Input: part model. Units: mm. Frame: model coordinates. A direction names the side the tool comes from. Round coordinates to 2 decimals unless told otherwise and drop trailing zeros. Order: outer loops, then holes, each group sorted by start corner. A loop starts at its lowest first (then second) coordinate and runs counter-clockwise, first axis right, second up. Notation, with made-up numbers: (71, 21) -> (130, 21) arc R17 cw to (130, 54) -> close; hole circle Ø3 at (-1.5, 43.5). An arc over 180 degrees is marked (long way). Use a Markdown table: item, result.
from build123d import *

# Parameters (mm, degrees)
SKETCH1_R           = 1.2
BOSS_EXTRUDE1_DEPTH = 8.7
CUT_EXTRUDE2_DEPTH  = 3
CUT_EXTRUDE3_DEPTH  = 3.8
CUT_EXTRUDE4_DEPTH  = 1.9
SKETCH5_W           = 1
SKETCH5_H           = 1.5
CUT_EXTRUDE5_DEPTH  = 3
FILLET1_R           = 1


with BuildPart() as part:
    # Sketch1 → Boss-Extrude1 (new body)
    with BuildSketch(Plane.XY):
        with BuildLine():
            Line((21.25, -19.25), (21.25, 19.25))
            ThreePointArc((21.25, 19.25), (20.664213562, 20.664213562), (19.25, 21.25))
            Line((19.25, 21.25), (-19.25, 21.25))
            ThreePointArc((-19.25, 21.25), (-20.664213562, 20.664213562), (-21.25, 19.25))
            Line((-21.25, 19.25), (-21.25, -19.25))
            ThreePointArc((-21.25, -19.25), (-20.664213562, -20.664213562), (-19.25, -21.25))
            Line((-19.25, -21.25), (19.25, -21.25))
            ThreePointArc((19.25, -21.25), (20.664213562, -20.664213562), (21.25, -19.25))
        make_face()
        with Locations(Location((-17, -17, 0), (0, 0, 180))):
            Circle(SKETCH1_R, mode=Mode.SUBTRACT)
        with Locations(Location((17, -17, 0), (0, 0, 180))):
            Circle(SKETCH1_R, mode=Mode.SUBTRACT)
        with Locations(Location((17, 17, 0), (0, 0, 180))):
            Circle(SKETCH1_R, mode=Mode.SUBTRACT)
        with Locations(Location((-17, 17, 0), (0, 0, 180))):
            Circle(SKETCH1_R, mode=Mode.SUBTRACT)
    extrude(amount=BOSS_EXTRUDE1_DEPTH)

    # Sketch2 → Cut-Extrude2 (cut)
    with BuildSketch(Plane(origin=(0, 0, 0), x_dir=(-1, 0, 0), z_dir=(0, 0, -1))):
        with BuildLine():
            Line((14.55, -19.25), (-14.55, -19.25))
            Line((-14.55, -19.25), (-14.55, -17))
            ThreePointArc((-14.55, -17), (-15.267588386, -15.267588386), (-17, -14.55))
            Line((-17, -14.55), (-19.25, -14.55))
            Line((-19.25, -14.55), (-19.25, 14.55))
            Line((-19.25, 14.55), (-17, 14.55))
            ThreePointArc((-17, 14.55), (-15.267588386, 15.267588386), (-14.55, 17))
            Line((-14.55, 17), (-14.55, 19.25))
            Line((-14.55, 19.25), (14.55, 19.25))
            Line((14.55, 19.25), (14.55, 17))
            ThreePointArc((14.55, 17), (15.267588386, 15.267588386), (17, 14.55))
            Line((17, 14.55), (19.25, 14.55))
            Line((19.25, 14.55), (19.25, -14.55))
            Line((19.25, -14.55), (17, -14.55))
            ThreePointArc((17, -14.55), (15.267588386, -15.267588386), (14.55, -17))
            Line((14.55, -17), (14.55, -19.25))
        make_face()
    extrude(amount=-CUT_EXTRUDE2_DEPTH, mode=Mode.SUBTRACT)

    # Sketch3 → Cut-Extrude3 (cut)
    with BuildSketch(Plane(origin=(0, 0, 3), x_dir=(-1, 0, 0), z_dir=(0, 0, -1))):
        with BuildLine():
            Line((-12.2, -6), (-12.2, 6))
            ThreePointArc((-12.2, 6), (-10.091168825, 11.091168825), (-5, 13.2))
            Line((-5, 13.2), (5, 13.2))
            ThreePointArc((5, 13.2), (10.091168825, 11.091168825), (12.2, 6))
            Line((12.2, 6), (12.2, -6))
            ThreePointArc((12.2, -6), (10.091168825, -11.091168825), (5, -13.2))
            Line((5, -13.2), (-5, -13.2))
            ThreePointArc((-5, -13.2), (-10.091168825, -11.091168825), (-12.2, -6))
        make_face()
    extrude(amount=-CUT_EXTRUDE3_DEPTH, mode=Mode.SUBTRACT)

    # Sketch4 → Cut-Extrude4 (cut)
    with BuildSketch(Plane.XY.offset(8.7)):
        with BuildLine():
            Line((21.25, 1.6), (7.173736823, 1.6))
            ThreePointArc((7.173736823, 1.6), (-7.35, 0), (7.173736823, -1.6))
            Line((7.173736823, -1.6), (21.25, -1.6))
            Line((21.25, -1.6), (21.25, 1.6))
        make_face()
    extrude(amount=-CUT_EXTRUDE4_DEPTH, mode=Mode.SUBTRACT)

    # Sketch5 → Cut-Extrude5 (cut)
    with BuildSketch(Plane(origin=(0, 0, 0), x_dir=(-1, 0, 0), z_dir=(0, 0, -1))):
        with Locations((-19.75, -10.3)):
            Rectangle(SKETCH5_W, SKETCH5_H)
    extrude(amount=-CUT_EXTRUDE5_DEPTH, mode=Mode.SUBTRACT)

    # Fillet1
    fillet1_edges = [part.edges().sort_by_distance(p)[0] for p in [
        (19.25, -11.05, 1.5),
        (19.25, -9.55, 1.5),
        (16.725, -1.6, 6.8),
        (16.725, 1.6, 6.8),
    ]]
    fillet(fillet1_edges, radius=FILLET1_R - 0.0001)  # a hair under: the kernel refuses the full size


solid = part.part
1) Cut plane B-B on z = 4.25. Return loops of the section in (x, y).
Results found:
| item | result |
|---|---|
| outline | (-21.25, -19.25) arc R2 ccw to (-19.25, -21.25) -> (19.25, -21.25) arc R2 ccw to (21.25, -19.25) -> (21.25, 19.25) arc R2 ccw to (19.25, 21.25) -> (-19.25, 21.25) arc R2 ccw to (-21.25, 19.25) -> close; hole circle Ø2.4 at (-17, -17); hole circle Ø2.4 at (-17, 17); hole (-12.2, -6) arc R7.2 ccw to (-5, -13.2) -> (5, -13.2) arc R7.2 ccw to (12.2, -6) -> (12.2, 6) arc R7.2 ccw to (5, 13.2) -> (-5, 13.2) arc R7.2 ccw to (-12.2, 6) -> close; hole circle Ø2.4 at (17, -17); hole circle Ø2.4 at (17, 17) |
2) Set-up query: faces 5 (the flat face through (13, -1.6, 8)), 6 (the cylindrical face through (17.26, 18.17, 4.29)), 7 (the flat face through (0, -19.25, 1)). Return all of +Z, -Z, +X, -X, +Y, -Y with unobstructed straight access to the full face (end or side cutting, diameter ignored); none if empty.
Results found:
| item | result |
|---|---|
| face 5 | +Z |
| face 6 | +Z, -Z |
| face 7 | -Z |
3) Line query: L1, parallel to Y at x = -17, z = 6.25; L2, parallel to X at y = 17, z = 2.5. Output: solid intervals per line, ascending. Write a range as [from, to].
Results found:
| item | result |
|---|---|
| L1 | y = [-21.25, -18.2], [-15.8, 15.8], [18.2, 21.25] |
| L2 | x = [-21.25, -18.2], [-15.8, -14.55], [14.55, 15.8], [18.2, 21.25] |
4) Pull-direction query (X, two-part tool) for faces 1 (the cylindrical face through (16.662, 1.315, 7.101)), 2 (the cylindrical face through (-20.65, 20.68, 4.29)), 3 (the flat face through (14.55, -18, 1)), 4 (the cylindrical face through (15.249, -15.287, 1.479)); classes: +X half, -X half, draft (parallel to the pull), parting line (faces both ways), or undercut.
Results found:
| item | result |
|---|---|
| face 1 | draft |
| face 2 | -X half |
| face 3 | undercut |
| face 4 | undercut |
5) Cut plane A-A on y = 0. Return loops of the section in (x, z), and give its area (3 significant figures).
Results found:
| item | result |
|---|---|
| outline | (-21.25, 0) -> (-19.25, 0) -> (-19.25, 3) -> (-12.2, 3) -> (-12.2, 6.8) -> (-7.35, 6.8) -> (-7.35, 8.7) -> (-21.25, 8.7) -> close; (12.2, 3) -> (19.25, 3) -> (19.25, 0) -> (21.25, 0) -> (21.25, 6.8) -> (12.2, 6.8) -> close |
| area | 107 mm² |
6) Cut plane C-C on x = -4.5. Return loops of the section in (y, z).
Results found:
| item | result |
|---|---|
| outline | (-21.25, 0) -> (-19.25, 0) -> (-19.25, 3) -> (-13.2, 3) -> (-13.2, 6.8) -> (-5.81, 6.8) -> (-5.81, 8.7) -> (-21.25, 8.7) -> close; (5.81, 6.8) -> (13.2, 6.8) -> (13.2, 3) -> (19.25, 3) -> (19.25, 0) -> (21.25, 0) -> (21.25, 8.7) -> (5.81, 8.7) -> close |
7) Cut plane D-D on y = -16.5. Return loops of the section in (x, z), and give its area (3 significant figures).
Results found:
| item | result |
|---|---|
| outline | (-21.25, 0) -> (-18.09, 0) -> (-18.09, 8.7) -> (-21.25, 8.7) -> close; (-15.91, 0) -> (-14.6, 0) -> (-14.6, 3) -> (14.6, 3) -> (14.6, 0) -> (15.91, 0) -> (15.91, 8.7) -> (-15.91, 8.7) -> close; (18.09, 0) -> (21.25, 0) -> (21.25, 8.7) -> (18.09, 8.7) -> close |
| area | 244 mm² |
8) Pin query (flat end, axial travel): pin 1 Ø12 at (x, y) = (0, 0) entering from +Z; pin 2 Ø5 at (x, y) = (-0.5, 14) entering from -Z. Return the tip coordinate at first contact, or that it passes through.
Results found:
| item | result |
|---|---|
| pin 1 | passes through |
| pin 2 | stops at z = 3 |
